Autodesk Inventor part; units mm, degrees
ref_plane "Work Plane1" through (0, 0, 1.7625) normal (0, 0, 1) x (1, 0, 0)
ref_plane "YZ Plane" through (0, 0, 0) normal (1, 0, 0) x (0, 1, 0)
ref_plane "XZ Plane" through (0, 0, 0) normal (0, 1, 0) x (-1, 0, 0)
sketch "Sketch1" plane through (0, 0, 0) normal (0, 0, 1) x (1, 0, 0)
  line L0 (176.5, -149) -> (-176.5, -149)
  line L1 (-176.5, -149) -> (-176.5, 149)
  line L2 (-176.5, 149) -> (176.5, 149)
  line L3 (176.5, 149) -> (176.5, -149)
  line L4 (176.5, -149) -> (-176.5, 149) construction
  line L5 (-176.5, -149) -> (176.5, 149) construction
  point P0 (0, 0)
  dimension "d0" = 353
  dimension "d1" = 298
extrude "Extrusion1" add sketch "Sketch1" along normal blind 4.7625
fillet "Fillet1" radius 4 4 edges at (-176.5, -149, 2.3813) (176.5, -149, 2.3813) (176.5, 149, 2.3813) (-176.5, 149, 2.3813)
sketch "Sketch2" plane through (0, 0, 4.7625) normal (0, 0, 1) x (1, 0, 0)
  arc A0 (-172.5, 149) -> (-176.5, 145) centre (-172.5, 145) ccw
  line L0 (-176.5, 145) -> (-176.5, -145)
  arc A1 (-176.5, -145) -> (-172.5, -149) centre (-172.5, -145) ccw
  line L1 (-172.5, -149) -> (172.5, -149)
  arc A2 (172.5, -149) -> (176.5, -145) centre (172.5, -145) ccw
  line L2 (176.5, -145) -> (176.5, 145)
  arc A3 (176.5, 145) -> (172.5, 149) centre (172.5, 145) ccw
  line L3 (172.5, 149) -> (-172.5, 149)
  arc A4 (-172.5, 148.5) -> (-176, 145) centre (-172.5, 145) ccw
  line L4 (-176, 145) -> (-176, -145)
  arc A5 (-176, -145) -> (-172.5, -148.5) centre (-172.5, -145) ccw
  line L5 (-172.5, -148.5) -> (172.5, -148.5)
  arc A6 (172.5, -148.5) -> (176, -145) centre (172.5, -145) ccw
  line L6 (176, -145) -> (176, 145)
  arc A7 (176, 145) -> (172.5, 148.5) centre (172.5, 145) ccw
  line L7 (172.5, 148.5) -> (-172.5, 148.5)
  point P0 (0, 0)
  dimension "d5" = 0.5
extrude "Extrusion2" cut sketch "Sketch2" against normal through all
sketch "Sketch3" plane through (0, 0, 0) normal (0, 0, -1) x (-1, 0, 0)
  arc A0 (-172.5, 148.5) -> (-176, 145) centre (-172.5, 145) ccw
  line L0 (-176, 145) -> (-176, -145)
  arc A1 (-176, -145) -> (-172.5, -148.5) centre (-172.5, -145) ccw
  line L1 (-172.5, -148.5) -> (172.5, -148.5)
  arc A2 (172.5, -148.5) -> (176, -145) centre (172.5, -145) ccw
  line L2 (176, -145) -> (176, 145)
  arc A3 (176, 145) -> (172.5, 148.5) centre (172.5, 145) ccw
  line L3 (172.5, 148.5) -> (-172.5, 148.5)
  arc A4 (-172.5, 160.5) -> (-188, 145) centre (-172.5, 145) ccw
  line L4 (-188, 145) -> (-188, -145)
  arc A5 (-188, -145) -> (-172.5, -160.5) centre (-172.5, -145) ccw
  line L5 (-172.5, -160.5) -> (172.5, -160.5)
  arc A6 (172.5, -160.5) -> (188, -145) centre (172.5, -145) ccw
  line L6 (188, -145) -> (188, 145)
  arc A7 (188, 145) -> (172.5, 160.5) centre (172.5, 145) ccw
  line L7 (172.5, 160.5) -> (-172.5, 160.5)
  point P0 (0, 0)
  dimension "d8" = 12
ref_plane "Work Plane1" through (0, 0, 1.7625) normal (0, 0, 1) x (1, 0, 0)
extrude "Extrusion3" add sketch "Sketch3" against normal up to surface (1.7625 mm away)
properties part number "Door Window" material "Polycarbonate, Smoke"
Here's how the part is built. I have some questions about the finished solid (model axes, mm). A direction names the side the tool comes from. Coordinates: 2 decimals unless noted, no trailing zeros. Loops run counter-clockwise (first coordinate to the right, second up) from the corner with the lowest first, then second, coordinate; pieces in that order, holes last.
1. Imagine slicing it at A-A, the plane y = -88. Please give me the cut outline in (x, z), and give its area (3 significant figures).
2. For faces 4 (the cylindrical face through (-183.34, -156.08, 0.87)), 5 (the flat face through (15, -154, 1.762)), which set-ups out of +Z, -Z, +X, -X, +Y, -Y let a thin tool reach every point of the face, with its end or its side?
3. For P1, Ø1.5, axis at x = -6, z = 3.5, coming from the +Y side; P2, Ø0.9, axis at y = -52, z = 2.5, coming from the -X side, each with a flat end and sliding along its axis, tell me the tip position at first contact or that it passes through.
4. Imagine slicing it at B-B, the plane x = -160. Please give me the cut outline in (y, z), and give its area (3 significant figures).
5. I need wall thicknesses on L1, parallel to X at y = 70, z = 3.65; L2, parallel to Y at x = 66, z = 4.25; L3, parallel to X at y = -146.5, z = 0.5. Which ranges of each line are inside material? Lowest first, please.
6. If we mould it in two halves opening along Y, with no side actions, what happens to faces 1 (the flat face through (-2, 2, 4.762)), 2 (the cylindrical face through (-183.58, 155.84, 0.87)), 3 (the cylindrical face through (183.58, -155.84, 0.87))? For each: pulls with the +Y half, pulls with the -Y half, needs draft (parallel to the pull), parting line crosses it, or undercut.
Taken from the geometry:
1. outline: (-188, 0) - (188, 0) - (188, 1.76) - (176, 1.76) - (176, 4.76) - (-176, 4.76) - (-176, 1.76) - (-188, 1.76) - close
1. area: 1,720 mm2
2. face 4: +Z, -Z, -X, -Y
2. face 5: +Z
3. P1: stops at y = 148.5
3. P2: stops at x = -176
4. outline: (-160.5, 0) - (160.5, 0) - (160.5, 1.76) - (148.5, 1.76) - (148.5, 4.76) - (-148.5, 4.76) - (-148.5, 1.76) - (-160.5, 1.76) - close
4. area: 1,460 mm2
5. L1: x = -176 to 176
5. L2: y = -148.5 to 148.5
5. L3: x = -187.93 to 187.93
6. face 1: needs draft
6. face 2: pulls with the +Y half
6. face 3: pulls with the -Y half
